Here's the drawing with two shaded views (mm, measured from the low corner). I have some questions. Coordinates: 2 decimals unless noted, no trailing zeros. Loops run counter-clockwise (first coordinate to the right, second up) from the corner with the lowest first, then second, coordinate; pieces in that order, holes last. Notation, with made-up numbers: (35.25, 23.25) -> (54.25, 23.25) arc R31 ccw to (54.25, 49.25) -> close; hole circle Ø5 at (39, -6). An arc over 180 degrees is marked (long way). Answer as a JSON object with one key per item and string values. Group by question number.
1) I need wall thicknesses on probe 1 along X at (y, z) = (1.3, 69.5); probe 2 along X at (y, z) = (2.7, 16.5); probe 3 along Z at (x, y) = (36.5, 1.4). Which ranges of each line are inside material? Lowest first, please. Write a range as [from, to].
2) I'm going to push flat-ended pins straight in: pin 1 (9 mm diameter, centred on x = 42.5, z = 69.5, fed in from +Y); pin 2 (1 mm diameter, centred on y = 2.5, z = 24.5, fed in from -X); pin 3 (3 mm diameter, centred on x = 40.5, y = 3, fed in from -Z). Where does each tip first touch, or does it pass through?
3) I want a section at A-A (z = 69.5). Write out the boundary of the cut face in (x, y).
4) I want a section at D-D (x = 73). Write out the boundary of the cut face in (y, z), then the cut area to 3 significant figures.
5) I want a section at B-B (x = 42.5). Write out the boundary of the cut face in (y, z).
6) I want a section at C-C (y = 2.9). Write out the boundary of the cut face in (x, z).
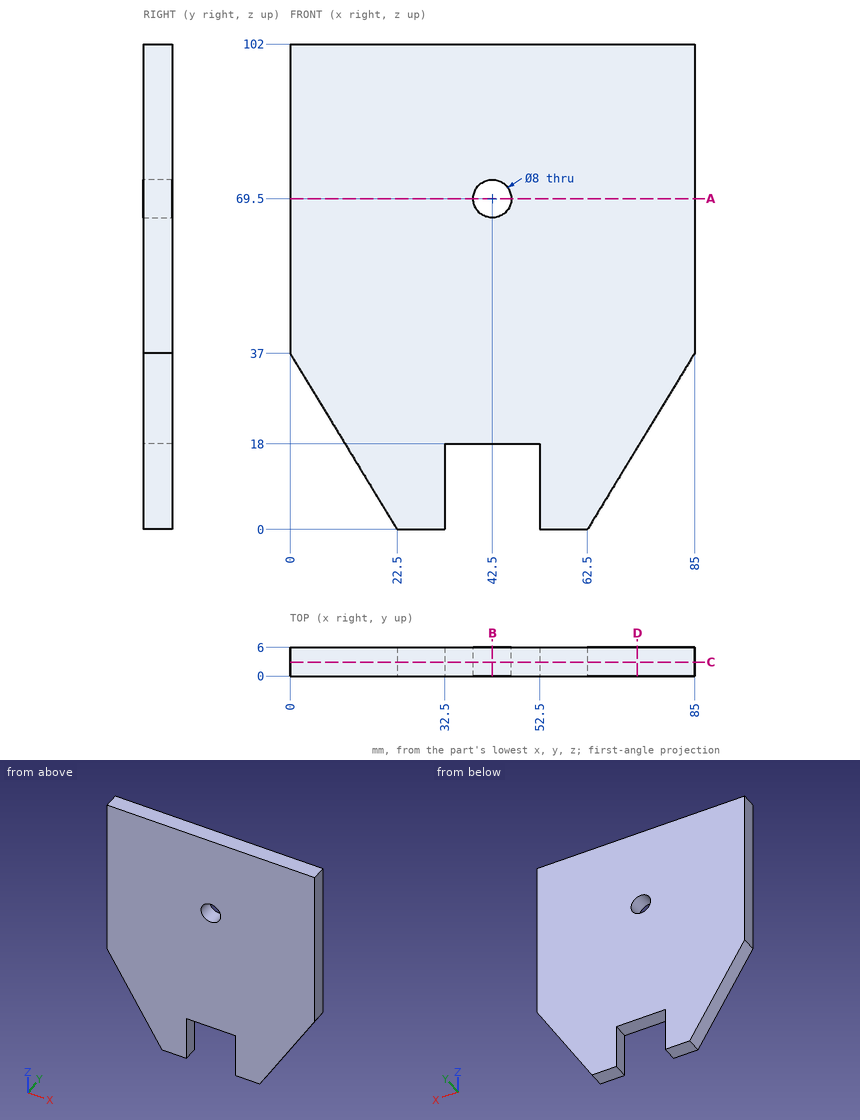
Determined:
{
 "1": {"probe 1": "[0, 38.5], [46.5, 85]", "probe 2": "[12.47, 32.5], [52.5, 72.53]", "probe 3": "[18, 102]"},
 "2": {"pin 1": "y = 6", "pin 2": "x = 7.3", "pin 3": "z = 18"},
 "3": {"outline": "(0, 0) -> (38.5, 0) -> (38.5, 6) -> (0, 6) -> close; (46.5, 0) -> (85, 0) -> (85, 6) -> (46.5, 6) -> close"},
 "4": {"outline": "(0, 17.27) -> (6, 17.27) -> (6, 102) -> (0, 102) -> close", "area": "508 mm^2"},
 "5": {"outline": "(0, 18) -> (6, 18) -> (6, 65.5) -> (0, 65.5) -> close; (0, 73.5) -> (6, 73.5) -> (6, 102) -> (0, 102) -> close"},
 "6": {"outline": "(0, 37) -> (22.5, 0) -> (32.5, 0) -> (32.5, 18) -> (52.5, 18) -> (52.5, 0) -> (62.5, 0) -> (85, 37) -> (85, 102) -> (0, 102) -> close; hole circle Ø8 at (42.5, 69.5)"}
}
